```python
from build123d import *

# Parameters (mm, degrees)
SKETCH2_R           = 8
SKETCH2_R_2         = 5.25
BOSS_EXTRUDE1_DEPTH = 10
BOSS_EXTRUDE2_DEPTH = 5
SKETCH4_R           = 1
CUT_EXTRUDE1_DEPTH  = 5


with BuildPart() as part:
    # Sketch2 → Boss-Extrude1 (new body)
    with BuildSketch(Plane(origin=(0, 0, 0), x_dir=(1, 0, 0), z_dir=(0, 1, 0))):
        with Locations(Location((0, 0, 0), (0, 0, 270))):
            Circle(SKETCH2_R)
        with Locations(Location((0, 0, 0), (0, 0, 270))):
            Circle(SKETCH2_R_2, mode=Mode.SUBTRACT)
    extrude(amount=BOSS_EXTRUDE1_DEPTH)

    # Sketch3 → Boss-Extrude2 (add)
    with BuildSketch(Plane(origin=(0, 10, 0), x_dir=(1, 0, 0), z_dir=(0, 1, 0))):
        with BuildLine():
            Line((0, 8), (-25, 5.901469298))
            ThreePointArc((-25, 5.901469298), (-30.901469298, 0), (-25, -5.901469298))
            Line((-25, -5.901469298), (0, -8))
            Line((0, -8), (25, -5.901469298))
            ThreePointArc((25, -5.901469298), (30.901469298, 0), (25, 5.901469298))
            Line((25, 5.901469298), (0, 8))
        make_face()
    extrude(amount=BOSS_EXTRUDE2_DEPTH)

    # Sketch4 → Cut-Extrude1 (cut)
    with BuildSketch(Plane(origin=(0, 15, 0), x_dir=(1, 0, 0), z_dir=(0, 1, 0))):
        with Locations(Location((-25, 0, 0), (0, 0, 270))):
            Circle(SKETCH4_R)
        with Locations(Location((25, 0, 0), (0, 0, 270))):
            Circle(SKETCH4_R)
    extrude(amount=-CUT_EXTRUDE1_DEPTH, mode=Mode.SUBTRACT)


solid = part.part
```
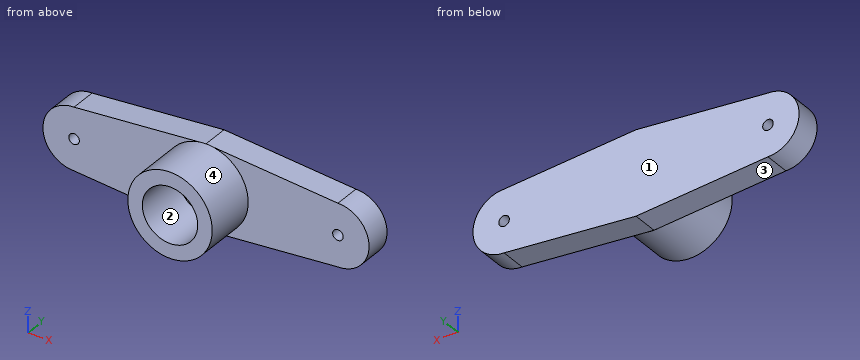
Could you check a few things on this model? Use its own coordinates, in mm. Face numbers are marked on the shaded views. Coordinates: 2 decimals unless noted, no trailing zeros. Loops run counter-clockwise (first coordinate to the right, second up) from the corner with the lowest first, then second, coordinate; pieces in that order, holes last. Notation, with made-up numbers: M 44,46 L 86,46 A26 ccw 86,84 Z; hole C 81.5,-18 d2. An arc over 180 degrees is marked long. Put each result on its own line as item: value. Start each with the question number.
(1) Thinking about a two-plate mould opening in Z: for the marked faces 1, 2, 3 and 4, which applies, pulls with the +Z half, pulls with the -Z half, needs draft (parallel to the pull), parting line crosses it, or undercut?
(2) Suppose I cut it at B-B on y = 11.5. Please give me the cut outline in (x, z).
(3) Suppose I cut it at A-A on z = 0. Please give me the cut outline in (x, y), then the cut area to 3 significant figures.
(4) Suppose I cut it at D-D on y = 6. Please give me the cut outline in (x, z), then the cut area to 3 significant figures.
(5) Will these pins go through, and if not, where does the flat tip stop? P1, Ø2, axis at y = 6.5, z = -4, coming from the -X side; P2, Ø1, axis at y = 3.5, z = 2.5, coming from the +X side; P3, Ø1, axis at x = -22, y = 10.5, coming from the +Z side; P4, Ø1.8, axis at x = -25, z = 0, coming from the +Y side.
(6) I need wall thicknesses on line 1 (X direction, y = 11.7, z = 0); line 2 (X direction, y = 2, z = 0); line 3 (Y direction, x = 15, z = -3.5). Which ranges of each line are inside material? Lowest first, please. Write a range as from..to.
(7) Suppose I cut it at C-C on z = 2.5. Please give me the cut outline in (x, y).
Solutions:
1. face 1: needs draft
1. face 2: undercut
1. face 3: pulls with the -Z half
1. face 4: parting line crosses it
2. outline: M -25,-5.9 L 0,-8 L 25,-5.9 A5.9 ccw 25,5.9 L 0,8 L -25,5.9 A5.9 ccw Z; hole C -25,0 d2; hole C 25,0 d2
3. outline: M -30.9,10 L -26,10 L -26,15 L -30.9,15 Z; M -24,10 L -8,10 L -8,0 L -5.25,0 L -5.25,10 L 5.25,10 L 5.25,0 L 8,0 L 8,10 L 24,10 L 24,15 L -24,15 Z; M 26,10 L 30.9,10 L 30.9,15 L 26,15 Z
3. area: 344 mm2
4. outline: C 0,0 d16; hole C 0,0 d10.5
4. area: 114 mm2
5. P1: stops at x = -7.42
5. P2: stops at x = 7.75
5. P3: stops at z = 6.2
5. P4: passes through
6. line 1: x = -30.9..-26, -24..24, 26..30.9
6. line 2: x = -8..-5.25, 5.25..8
6. line 3: y = 10..15
7. outline: M -30.35,10 L -7.6,10 L -7.6,0 L -4.62,0 L -4.62,10 L 4.62,10 L 4.62,0 L 7.6,0 L 7.6,10 L 30.35,10 L 30.35,15 L -30.35,15 Z
